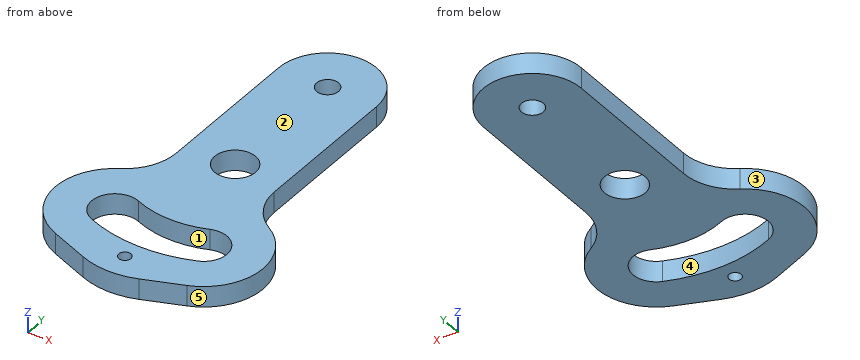
from build123d import *

# Parameters (mm, degrees)
SKETCH_1_R      = 7.9
SKETCH_1_R_2    = 4.25
SKETCH_1_R_3    = 2.35
EXTRUDE_1_DEPTH = 8
FILLET_1_R      = 30


with BuildPart() as part:
    # Эскиз1 → Бобышка-Вытянуть1 (new body)
    with BuildSketch(Plane.XY):
        with BuildLine():
            Line((-19, 114), (-19, 56.432557211))
            ThreePointArc((-19, 56.432557211), (-21.643532577, 46.495100866), (-28.875303859, 39.18464348))
            ThreePointArc((-28.875303859, 39.18464348), (-40.157482483, 17.500808258), (-25.546486414, -2.094983595))
            Line((-25.546486414, -2.094983595), (0, -12))
            Line((0, -12), (25.546486414, -2.094983595))
            ThreePointArc((25.546486414, -2.094983595), (40.157482483, 17.500808258), (28.875303859, 39.18464348))
            ThreePointArc((28.875303859, 39.18464348), (21.643532577, 46.495100866), (19, 56.432557211))
            Line((19, 56.432557211), (19, 114))
            ThreePointArc((19, 114), (0, 133), (-19, 114))
        make_face()
        with Locations((0, 62)):
            Circle(SKETCH_1_R, mode=Mode.SUBTRACT)
        with Locations((0, 114)):
            Circle(SKETCH_1_R_2, mode=Mode.SUBTRACT)
        Circle(SKETCH_1_R_3, mode=Mode.SUBTRACT)
        with BuildLine():
            ThreePointArc((-20.603362638, 11.004887999), (0, 7), (20.603362638, 11.004887999))
            ThreePointArc((20.603362638, 11.004887999), (25.576557988, 22.721002031), (13.860443956, 27.694197381))
            ThreePointArc((13.860443956, 27.694197381), (0, 25), (-13.860443956, 27.694197381))
            ThreePointArc((-13.860443956, 27.694197381), (-25.576557988, 22.721002031), (-20.603362638, 11.004887999))
        make_face(mode=Mode.SUBTRACT)
    extrude(amount=EXTRUDE_1_DEPTH)

    # Скругление1
    fillet_1_edges = [part.edges().sort_by_distance(p)[0] for p in [
        (0, -12, 4),
    ]]
    fillet(fillet_1_edges, radius=FILLET_1_R)


solid = part.part
Source: CAD feature listing. Evaluate the final solid. Frame: model axes, mm. Face numbers are marked on the shaded views. A direction names the side the tool comes from. Round coordinates to 2 decimals unless told otherwise and drop trailing zeros. Loops run counter-clockwise (first coordinate to the right, second up) from the corner with the lowest first, then second, coordinate; pieces in that order, holes last.
Q1. Mould query, pull axis Y, two halves, no side actions, for the marked faces 1, 2 and 3. Classes: pulls with the +Y half, pulls with the -Y half, needs draft (parallel to the pull), parting line crosses it, or undercut.
Q2. Ray query, line 1 (Y direction, x = -5, z = 4.5); line 2 (X direction, y = 113.5, z = 0.5); line 3 (X direction, y = 24.5, z = 1.5). Return the intervals inside material, ascending.
Q3. Section A-A, the plane x = 0. Return loops of the section in (y, z).
Q4. First-contact query: P1, Ø5.5, axis at x = 0, y = 0, coming from the +Z side; P2, Ø2, axis at x = 4.5, z = 4, coming from the +Y side; P3, Ø2.5, axis at y = 98.5, z = 3.5, coming from the +X side; P4, Ø2.5, axis at y = 88.5, z = 3, coming from the -X side. Flat tips, straight axial feed; report the tip coordinate or a pass-through.
Q5. Section D-D, the plane x = 24. Return loops of the section in (y, z), plus the area to 3 significant figures.
Q6. Access query for the marked faces 4 and 5. Directions: +Z, -Z, +X, -X, +Y, -Y. A direction counts if a zero-diameter tool reaches every point of the face in a straight line with its end or side. Return the directions, or none.
Q7. Section C-C, the plane z = 6. Return loops of the section in (x, y), plus the area to 3 significant figures.
Q8. Section B-B, the plane y = 62. Return loops of the section in (x, z).
Solutions:
1. face 1: undercut
1. face 2: needs draft
1. face 3: parting line crosses it
2. line 1: y = -9.4 to 7.23, 25.34 to 55.88, 68.12 to 132.33
2. line 2: x = -19 to -4.22, 4.22 to 19
2. line 3: x = -39.65 to -24.61, 24.61 to 39.65
3. outline: (-9.82, 0) - (-2.35, 0) - (-2.35, 8) - (-9.82, 8) - close; (2.35, 0) - (7, 0) - (7, 8) - (2.35, 8) - close; (25, 0) - (54.1, 0) - (54.1, 8) - (25, 8) - close; (69.9, 0) - (109.75, 0) - (109.75, 8) - (69.9, 8) - close; (118.25, 0) - (133, 0) - (133, 8) - (118.25, 8) - close
4. P1: stops at z = 8
4. P2: stops at y = 132.67
4. P3: stops at x = 19
4. P4: stops at x = -19
5. outline: (-2.69, 0) - (13.42, 0) - (13.42, 8) - (-2.69, 8) - close; (25.28, 0) - (43.2, 0) - (43.2, 8) - (25.28, 8) - close
5. area: 272 mm2
6. face 4: +Z, -Z
6. face 5: +Z, -Z, +X
7. outline: (-28.88, 39.18) arc R23 ccw to (-25.55, -2.09) - (-10.85, -7.8) arc R30 ccw to (10.85, -7.8) - (25.55, -2.09) arc R23 ccw to (28.88, 39.18) arc R20 cw to (19, 56.43) - (19, 114) arc R19 ccw to (-19, 114) - (-19, 56.43) arc R20 cw to start; hole (-20.6, 11) arc R55 ccw to (20.6, 11) arc R9 ccw to (13.86, 27.69) arc R37 cw to (-13.86, 27.69) arc R9 ccw to start; hole circle Ø15.8 at (0, 62); hole circle Ø8.5 at (0, 114); hole circle Ø4.7 at (0, 0)
7. area: 5,600 mm2
8. outline: (-19, 0) - (-7.9, 0) - (-7.9, 8) - (-19, 8) - close; (7.9, 0) - (19, 0) - (19, 8) - (7.9, 8) - close
